Verification items for the finished model (mm, model axes). Face numbers are marked on the shaded views. A direction names the side the tool comes from. Coordinates: 2 decimals unless noted, no trailing zeros. Order: outer loops, then holes, each group sorted by start corner. A loop starts at its lowest first (then second) coordinate and runs counter-clockwise, first axis right, second up.
Q1. Cross-section at C-C, the plane y = -7. Record the boundary of the cut face in (x, z) (3 decimals).
Q2. Set-up check for the marked faces 4, 5 and 6: record each of +Z, -Z, +X, -X, +Y, -Y from which the full face is reachable in a straight line by a thin tool's end or side.
Q3. Cross-section at B-B, the plane x = 8. Record the boundary of the cut face in (y, z), and give its area (3 significant figures).
Q4. Draft check along Y on the marked faces 1, 2 and 3. Enter one of: pulls with the +Y half, pulls with the -Y half, needs draft (parallel to the pull), parting line crosses it, or undercut.
Q5. Cross-section at D-D, the plane z = 0. Record the boundary of the cut face in (x, y) (3 decimals), and give its area (3 significant figures).
Q6. Depth check by flat-ended pin: P1, Ø16, axis at x = -11.5, z = 48.5, coming from the +Y side; P2, Ø23, axis at x = -37, y = 17, coming from the -Z side; P3, Ø5.5, axis at x = 0, z = 0, coming from the -Y side. Enter the tip coordinate at first touch or a pass-through.
Q7. Thickness scan on line 1 (Z direction, x = 0, y = -6.5) (3 decimals); line 2 (Y direction, x = -14, z = 12); line 3 (Z direction, x = 10.5, y = 5.5). Record the ranges inside material, lowest first.
Q8. Cross-section at A-A, the plane z = 67. Record the boundary of the cut face in (x, y), and give its area (3 significant figures).
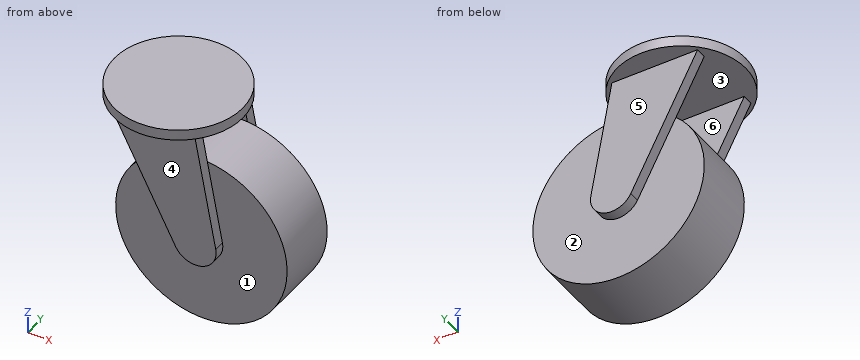
from build123d import *

# Parameters (mm, degrees)
F0_R     = 50.8
F0_R_2   = 3.175
F1_DEPTH = 19.05
F3_R     = 38.1
F4_DEPTH = 6.35
F6_DEPTH = 6.35


# Not quite as in the source:
# - a pattern or mirror of a feature is missing from the dataset's text; its kind, count and spacing are read off the source's solid


with BuildPart() as f1:
    # F0 (on Front) → F1 (new body, symmetric)
    with BuildSketch(Plane.XZ):
        Circle(F0_R)
        Circle(F0_R_2, mode=Mode.SUBTRACT)
    extrude(amount=F1_DEPTH, both=True)



with BuildPart() as f4:
    # F3 (on offset) → F4 (new body)
    with BuildSketch(Plane.XY.offset(76.2)):
        with Locations((-25.4, 0)):
            Circle(F3_R)
    extrude(amount=-F4_DEPTH)


with BuildPart() as f1_1:
    add(f1.part)

    add(f4.part)  # F6 merges F4
    # F5 (on face) → F6 (join)
    with BuildSketch(Plane(origin=(0, 19.05, 0), x_dir=(-1, 0, 0), z_dir=(0, 1, 0))):
        with BuildLine():
            Line((0, 69.85), (-12.4883185087, 2.3090909091))
            ThreePointArc((-12.4883185087, 2.3090909091), (-4.1396882106, -12.0063725379), (11.2576825912, -5.8783146118))
            Line((11.2576825912, -5.8783146118), (50.8, 69.85))
            Line((50.8, 69.85), (0, 69.85))
        make_face()
    f6 = extrude(amount=F6_DEPTH)

    # F6_copies: F6 across plane
    add(f6.mirror(Plane(origin=(0, 0, 0), x_dir=(0, 0, -1), z_dir=(0, -1, 0))))


solid = f1_1.part
Check values:
1. outline: (-62.851, 69.85) - (12.051, 69.85) - (12.051, 76.2) - (-62.851, 76.2) - close; circle Ø101.6 at (0, 0); hole circle Ø6.35 at (0, 0)
2. face 4: -Z, +X, -X, -Y
2. face 5: -Z, +X, -X, +Y
2. face 6: -X
3. outline: (-25.4, -9.86) - (-19.05, -9.86) - (-19.05, -50.17) - (19.05, -50.17) - (19.05, -9.86) - (25.4, -9.86) - (25.4, 26.58) - (19.05, 26.58) - (19.05, 50.17) - (-19.05, 50.17) - (-19.05, 26.58) - (-25.4, 26.58) - close; (-18.33, 69.85) - (18.33, 69.85) - (18.33, 76.2) - (-18.33, 76.2) - close
3. area: 4,520 mm2
4. face 1: pulls with the -Y half
4. face 2: pulls with the +Y half
4. face 3: undercut
5. outline: (-50.8, -19.05) - (-14.327, -19.05) - (-14.327, -25.4) - (12.7, -25.4) - (12.7, -19.05) - (50.8, -19.05) - (50.8, 19.05) - (12.7, 19.05) - (12.7, 25.4) - (-14.327, 25.4) - (-14.327, 19.05) - (-50.8, 19.05) - close; hole (-3.175, -19.05) - (3.175, -19.05) - (3.175, 19.05) - (-3.175, 19.05) - close
5. area: 3,970 mm2
6. P1: stops at y = 25.4
6. P2: stops at z = -43.94
6. P3: stops at y = -25.4
7. line 1: z = -50.8 to -3.175, 3.175 to 50.8, 69.85 to 76.2
7. line 2: y = -25.4 to 25.4
7. line 3: z = -49.7 to 49.7, 69.85 to 76.2
8. outline: (-49.31, -25.4) - (0.53, -25.4) - (0.53, -19.05) - (-49.31, -19.05) - close; (-49.31, 19.05) - (0.53, 19.05) - (0.53, 25.4) - (-49.31, 25.4) - close
8. area: 633 mm2
